Source: CAD feature listing. Evaluate the final solid. Frame: model axes, mm. Face numbers are marked on the shaded views. A direction names the side the tool comes from. Coordinates: 2 decimals unless noted, no trailing zeros. Order: outer loops, then holes, each group sorted by start corner. A loop starts at its lowest first (then second) coordinate and runs counter-clockwise, first axis right, second up. Notation, with made-up numbers: (87.25, -19) - (105.25, -19) arc R22 cw to (105.25, 15) - close; hole circle Ø5 at (74.25, -28). An arc over 180 degrees is marked (long way). One line per question, with ' | ' between items. Start each with the question number.
(1) Section C-C (z = -2). Return the cut outline in (x, y).
(2) Contact query for flat-ended pins moving along their axis: P1, Ø2, axis at x = 1.5, z = 26, coming from the +Y side (3 decimals); P2, Ø0.5, axis at x = -11.5, z = 2, coming from the +Y side; P3, Ø1.3, axis at x = -11, z = 1, coming from the -Y side. Output: stop coordinate, or through.
(3) Section B-B (x = 0). Return the cut outline in (y, z) (3 decimals).
(4) Section D-D (y = 3.75). Return the cut outline in (x, z), then the cut area to 3 significant figures.
(5) Line query: line 1 along Z through (x, y) = (-2.75, 5.25); line 2 along Z through (x, y) = (-2.25, 1.25); line 3 along Y through (x, z) = (2, -1.5). Output: solid intervals per line, ascending.
(6) Access query for the marked faces 1, 2 and 3. Directions: +Z, -Z, +X, -X, +Y, -Y. A direction counts if a zero-diameter tool reaches every point of the face in a straight line with its end or side. Return the directions, or none.
(7) Section A-A (y = 0). Return the cut outline in (x, z) (3 decimals).
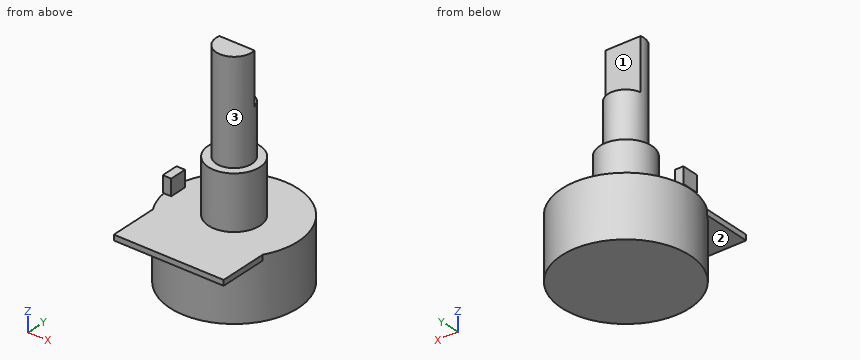
from build123d import *

# Parameters (mm, degrees)
CROQUIS2_W                 = 1.57
CROQUIS2_H                 = 3.2
SALIENTE_EXTRUIR1_DEPTH    = 3
SALIENTE_EXTRUIR2_DEPTH    = 1
CROQUIS4_W                 = 9.53
CROQUIS4_H                 = 2.67
CORTAR_EXTRUIR1_DEPTH      = 12.9
CORTAR_EXTRUIR1_DEPTH_BACK = 12.98


with BuildPart() as part:
    # Croquis1 → Revolución2 (revolve)
    with BuildSketch(Plane(origin=(0, 0, 0), x_dir=(0, 0, -1), z_dir=(1, 0, 0))):
        Polygon((0, 0), (11.3, 0), (11.3, 11.9), (0, 11.9), (0, 4.8), (-9.93, 4.8), (-9.93, 3.315), (-28.8, 3.315), (-28.8, 0), align=None)
    revolve(axis=Axis((0, 0, 28.8), (0, 0, -1)))

    # Croquis2 → Saliente-Extruir1 (add)
    with BuildSketch(Plane.XY):
        with Locations((-11.195, 0)):
            Rectangle(CROQUIS2_W, CROQUIS2_H)
    extrude(amount=SALIENTE_EXTRUIR1_DEPTH)

    # Croquis3 → Saliente-Extruir2 (add)
    with BuildSketch(Plane.XY):
        with BuildLine():
            Line((-10.2, -15.2), (10.2, -15.2))
            Line((10.2, -15.2), (10.2, -6.129437168))
            ThreePointArc((10.2, -6.129437168), (0, -11.9), (-10.2, -6.129437168))
            Line((-10.2, -6.129437168), (-10.2, -15.2))
        make_face()
    extrude(amount=-SALIENTE_EXTRUIR2_DEPTH)

    # Croquis4 → Cortar-Extruir1 (cut, two sides)
    with BuildSketch(Plane(origin=(0, 0, 0), x_dir=(0, 0, -1), z_dir=(1, 0, 0))) as cortar_extruir1_sk:
        with Locations((-24.035, 1.98)):
            Rectangle(CROQUIS4_W, CROQUIS4_H)
    extrude(amount=CORTAR_EXTRUIR1_DEPTH, mode=Mode.SUBTRACT)
    extrude(cortar_extruir1_sk.sketch, amount=-CORTAR_EXTRUIR1_DEPTH_BACK, mode=Mode.SUBTRACT)


solid = part.part
Response values:
1) outline: circle Ø23.8 at (0, 0)
2) P1: stops at y = 0.645 | P2: stops at y = 1.6 | P3: stops at y = -1.6
3) outline: (-15.2, -1) - (-11.9, -1) - (-11.9, -11.3) - (11.9, -11.3) - (11.9, 0) - (4.8, 0) - (4.8, 9.93) - (3.315, 9.93) - (3.315, 19.27) - (0.645, 19.27) - (0.645, 28.8) - (-3.315, 28.8) - (-3.315, 9.93) - (-4.8, 9.93) - (-4.8, 0) - (-15.2, 0) - close
4) outline: (-11.29, -11.3) - (11.29, -11.3) - (11.29, 0) - (3, 0) - (3, 9.93) - (-3, 9.93) - (-3, 0) - (-11.29, 0) - close | area: 315 mm²
5) line 1: z = -11.3 to 0 | line 2: z = -11.3 to 19.27 | line 3: y = -11.73 to 11.73
6) face 1: +Z, +X, -X, +Y | face 2: -Z, -Y | face 3: +Z
7) outline: (-11.98, 0) - (-11.9, 0) - (-11.9, -11.3) - (11.9, -11.3) - (11.9, 0) - (4.8, 0) - (4.8, 9.93) - (3.315, 9.93) - (3.315, 28.8) - (-3.315, 28.8) - (-3.315, 9.93) - (-4.8, 9.93) - (-4.8, 0) - (-10.41, 0) - (-10.41, 3) - (-11.98, 3) - close
